Check sheet for the modelled part. Datum: model origin and axes. Units: mm. A direction names the side the tool comes from. Give positions to 0.01 mm unless a question says otherwise; leave off trailing zeros. Write each loop counter-clockwise with the first axis right and the second up, starting at its lowest first coordinate (ties: lowest second). Pieces come first, ordered by that corner, then holes. Notation, with made-up numbers: M 72,63.5 L 100,63.5 A15 cw 100,76.5 Z; hole C -13,36.5 d10. An arc over 180 degrees is marked long. Use CSV: the item, a comma, the result in double quotes. Start each with the question number.
1. Scan lines: line 1 (Y direction, x = 12.5, z = 28.2) (3 decimals); line 2 (Y direction, x = 12.5, z = 29.55); line 3 (X direction, y = 10.5, z = 3.5). Record each from-to range of solid material in increasing order.
2. Depth check by flat-ended pin: P1, Ø1.8, axis at x = -14.5, y = 8, coming from the +Z side; P2, Ø1, axis at x = -4, y = -2.5, coming from the -Z side; P3, Ø1.8, axis at x = 12.365, y = 0, coming from the -Z side. Enter the tip coordinate at first touch or a pass-through.
3. Mould release check, pull along Y, two halves, no side actions. Record for faces 1 (the face through (3, 9.365, 1)), 2 (the face through (22.615, 0, 14)), 3 (the face through (15.5, -0.1, 30.7)), 4 (the face through (3, -9.365, 1)): +Y half, -Y half, draft (parallel to the pull), parting line (faces both ways), or undercut.
4. Cross-section at A-A, the plane x = -8.5. Enter the section's corners in (y, z) (3 decimals), and give its area (3 significant figures).
5. Access from +Z, -Z, +X, -X, +Y, -Y to the whole of each face (thin tool, end or side, straight path). Record for faces 5 (the face through (-0.75, 0.15, -2.4)), 6 (the face through (-21.615, 0, -1)), 7 (the face through (-9, -8, 30.5)), 8 (the face through (11, 0, 29)).
6. Cross-section at B-B, the plane x = 12.5. Enter the section's corners in (y, z) (3 decimals).
from build123d import *

# Parameters (mm, degrees)
SKETCH_1_W          = 45.23
SKETCH_1_H          = 24.73
EXTRUDE_1_DEPTH     = 29
FILLET_1_R          = 2
SKETCH_2_R          = 3
EXTRUDE_2_DEPTH     = 3.4
SKETCH_3_R          = 1.5
CUT_EXTRUDE_1_DEPTH = 6
SKETCH_4_W          = 25.725975672
SKETCH_4_H          = 22.73
EXTRUDE_3_DEPTH     = 1.5
SKETCH_5_R          = 0.5
CUT_EXTRUDE_2_DEPTH = 1.5
CUT_EXTRUDE_3_DEPTH = 1.5
EXTRUDE_START       = 1.5
EXTRUDE_4_DEPTH     = 1.5
SKETCH_21_W         = 21.4387918
SKETCH_21_H         = 22.73
EXTRUDE_11_DEPTH    = 1.5
CUT_EXTRUDE_START   = -1.5
SKETCH_23_R         = 0.5
CUT_EXTRUDE_4_DEPTH = 1.5
SKETCH_24_W         = 18.4387918
SKETCH_24_H         = 18.73
EXTRUDE_12_DEPTH    = 1.5
FILLET_2_R          = 2
SKETCH_25_R         = 3
EXTRUDE_13_DEPTH    = 4.1
SKETCH_26_R         = 1.5
CUT_EXTRUDE_5_DEPTH = 4.1
SKETCH_27_W         = 4
SKETCH_27_H         = 18.73
CUT_EXTRUDE_6_DEPTH = 3


with BuildPart() as part:
    # 草图1 → 凸台-拉伸1 (new body)
    with BuildSketch(Plane.XY):
        Rectangle(SKETCH_1_W, SKETCH_1_H)
    extrude(amount=EXTRUDE_1_DEPTH)

    # 圆角1
    fillet_1_edges = [part.edges().sort_by_distance(p)[0] for p in [
        (22.615, -12.365, 14.5),
        (-22.615, -12.365, 14.5),
        (-22.615, 12.365, 14.5),
        (22.615, 12.365, 14.5),
    ]]
    fillet(fillet_1_edges, radius=FILLET_1_R)

    # 草图2 → 凸台-拉伸2 (add)
    with BuildSketch(Plane.XY.offset(29)):
        with Locations(Location((12.5, 0, 0), (0, 0, 180))):
            Circle(SKETCH_2_R)
    extrude(amount=EXTRUDE_2_DEPTH)

    # 草图3 → 切除-拉伸1 (cut)
    with BuildSketch(Plane.XY.offset(32.4)):
        with Locations((12.5, 0)):
            Circle(SKETCH_3_R)
    extrude(amount=-CUT_EXTRUDE_1_DEPTH, mode=Mode.SUBTRACT)

    # 草图4 → 凸台-拉伸3 (add)
    with BuildSketch(Plane.XY.offset(29)):
        with Locations((-8.752012164, 0)):
            Rectangle(SKETCH_4_W, SKETCH_4_H)
    extrude(amount=EXTRUDE_3_DEPTH)

    # 草图5 → 切除-拉伸2 (cut)
    with BuildSketch(Plane.XY.offset(30.5)):
        with Locations((-21.615, 11.365)):
            Circle(SKETCH_5_R)
        with Locations((4.110975672, 11.365)):
            Circle(SKETCH_5_R)
        with Locations((-21.615, -11.365)):
            Circle(SKETCH_5_R)
        with Locations((4.110975672, -11.365)):
            Circle(SKETCH_5_R)
    extrude(amount=-CUT_EXTRUDE_2_DEPTH, mode=Mode.SUBTRACT)

    # 草图6 → 切除-拉伸3 (cut)
    with BuildSketch(Plane.XY.offset(30.5)):
        with BuildLine():
            Line((4.110975672, -8.580458661), (4.110975672, 8.580458661))
            ThreePointArc((4.110975672, 8.580458661), (0.5, 0), (4.110975672, -8.580458661))
        make_face()
    extrude(amount=-CUT_EXTRUDE_3_DEPTH, mode=Mode.SUBTRACT)

    # 草图7 → 凸台-拉伸4 (add)
    with BuildSketch(Plane.XY.offset(30.5).offset(EXTRUDE_START)):
        with BuildLine():
            Line((-21.615, 5.365), (1.766092277, 5.365))
            ThreePointArc((1.766092277, 5.365), (0.5, 0), (1.766092277, -5.365))
            Line((1.766092277, -5.365), (-21.615, -5.365))
            Line((-21.615, -5.365), (-21.615, 5.365))
        make_face()
    extrude(amount=-EXTRUDE_4_DEPTH)

    # 草图21 → 凸台-拉伸11 (add)
    with BuildSketch(Plane(origin=(-20.629587366, 0.959657155, 0), x_dir=(-1, 0, 0), z_dir=(0, 0, -1))):
        with Locations((-9.733983266, -0.959657155)):
            Rectangle(SKETCH_21_W, SKETCH_21_H)
    extrude(amount=EXTRUDE_11_DEPTH)

    # 草图23 → 切除-拉伸4 (cut)
    with BuildSketch(Plane(origin=(-20.629587366, 0.959657155, -1.5), x_dir=(-1, 0, 0), z_dir=(0, 0, -1)).offset(CUT_EXTRUDE_START)):
        with Locations((-20.453379166, 10.405342845)):
            Circle(SKETCH_23_R)
        with Locations((0.985412634, 10.405342845)):
            Circle(SKETCH_23_R)
        with Locations((-20.453379166, -12.324657155)):
            Circle(SKETCH_23_R)
        with Locations((0.985412634, -12.324657155)):
            Circle(SKETCH_23_R)
    extrude(amount=CUT_EXTRUDE_4_DEPTH, mode=Mode.SUBTRACT)

    # 草图24 → 凸台-拉伸12 (add)
    with BuildSketch(Plane(origin=(0, 0, -1.5), x_dir=(-1, 0, 0), z_dir=(0, 0, -1))):
        with Locations((9.3956041, 0)):
            Rectangle(SKETCH_24_W, SKETCH_24_H)
    extrude(amount=EXTRUDE_12_DEPTH)

    # 圆角2
    fillet_2_edges = [part.edges().sort_by_distance(p)[0] for p in [
        (-0.1762082, 0, -3),
    ]]
    fillet(fillet_2_edges, radius=FILLET_2_R)

    # 草图25 → 凸台-拉伸13 (add)
    with BuildSketch(Plane(origin=(0, 0, 0), x_dir=(-1, 0, 0), z_dir=(0, 0, -1))):
        with Locations((-12.365, 0)):
            Circle(SKETCH_25_R)
    extrude(amount=EXTRUDE_13_DEPTH)

    # 草图26 → 切除-拉伸5 (cut)
    with BuildSketch(Plane(origin=(0, 0, -4.1), x_dir=(-1, 0, 0), z_dir=(0, 0, -1))):
        with Locations((-12.365, 0)):
            Circle(SKETCH_26_R)
    extrude(amount=-CUT_EXTRUDE_5_DEPTH, mode=Mode.SUBTRACT)

    # 草图27 → 切除-拉伸6 (cut)
    with BuildSketch(Plane(origin=(0, 0, 0), x_dir=(-1, 0, 0), z_dir=(0, 0, -1))):
        with Locations((-2.8237918, 0)):
            Rectangle(SKETCH_27_W, SKETCH_27_H)
    extrude(amount=-CUT_EXTRUDE_6_DEPTH, mode=Mode.SUBTRACT)


solid = part.part
Worked answers:
1,line 1,"y = -12.365 to -1.5, 1.5 to 12.365"
1,line 2,"y = -3 to -1.5, 1.5 to 3"
1,line 3,"x = -22.61 to 22.61"
2,P1,"stops at z = 30.5"
2,P2,"stops at z = -3"
2,P3,"stops at z = 0"
3,face 1,"undercut"
3,face 2,"draft"
3,face 3,"parting line"
3,face 4,"undercut"
4,outline,"M -12.365,0 L -11.365,0 L -11.365,-1.5 L -9.365,-1.5 L -9.365,-3 L 9.365,-3 L 9.365,-1.5 L 11.365,-1.5 L 11.365,0 L 12.365,0 L 12.365,29 L 11.365,29 L 11.365,30.5 L 5.365,30.5 L 5.365,32 L -5.365,32 L -5.365,30.5 L -11.365,30.5 L -11.365,29 L -12.365,29 Z"
4,area,"830 mm^2"
5,face 5,"-Z, +Y, -Y"
5,face 6,"-Z, -X, +Y, -Y"
5,face 7,"+Z, +X, -X, -Y"
5,face 8,"+Z"
6,outline,"M -12.365,0 L -2.997,0 L -2.997,-4.1 L -1.494,-4.1 L -1.494,0 L 1.494,0 L 1.494,-4.1 L 2.997,-4.1 L 2.997,0 L 12.365,0 L 12.365,29 L 3,29 L 3,32.4 L 1.5,32.4 L 1.5,26.4 L -1.5,26.4 L -1.5,32.4 L -3,32.4 L -3,29 L -12.365,29 Z"
